```python
from build123d import *

# Parameters (mm, degrees)
SKETCH046_R     = 2.5
PAD023_DEPTH    = 2.5
SKETCH047_R     = 5
PAD024_DEPTH    = 3
FILLET003_R     = 1.5
SKETCH049_R     = 2.5
PAD025_DEPTH    = 4
SKETCH050_R     = 1.5
POCKET026_DEPTH = 4
SKETCH091_W     = 4
SKETCH091_H     = 4
SKETCH091_W_2   = 3
SKETCH091_H_2   = 3
PAD057_DEPTH    = 0.2


with BuildPart() as part:
    # Sketch046 → Pad023 (new body)
    with BuildSketch(Plane(origin=(0, 0, 30), x_dir=(1, 0, 0), z_dir=(0, 0, -1))):
        with Locations((101, 55)):
            Circle(SKETCH046_R)
    extrude(amount=-PAD023_DEPTH)

    # Sketch047 (on Face3 of Pad023) → Pad024 (join)
    with BuildSketch(Plane.XY.offset(32.5)):
        with Locations((101, -55)):
            Circle(SKETCH047_R)
    extrude(amount=PAD024_DEPTH)

    # Fillet003
    fillet003_edges = [part.edges().sort_by_distance(p)[0] for p in [
        (96, -55, 35.5),
    ]]
    fillet(fillet003_edges, radius=FILLET003_R)

    # Sketch049 → Pad025 (join)
    with BuildSketch(Plane(origin=(0, 0, 30), x_dir=(1, 0, 0), z_dir=(0, 0, -1))):
        with Locations((101, 55)):
            Circle(SKETCH049_R)
    extrude(amount=PAD025_DEPTH)

    # Sketch050 (on Face17 of Pad025) → Pocket026 (cut)
    with BuildSketch(Plane(origin=(0, 0, 26), x_dir=(1, 0, 0), z_dir=(0, 0, -1))):
        with Locations((101, 55)):
            Circle(SKETCH050_R)
    extrude(amount=-POCKET026_DEPTH, mode=Mode.SUBTRACT)


with BuildPart() as part_1:
    # Body002 placement: moved
    add(part.part.moved(Location((75, 0, 0))))

    # Sketch091 (on Face4 of Clone005) → Pad057 (new body)
    with BuildSketch(Plane(origin=(75, 0, 35.5), x_dir=(1, 0, 0), z_dir=(0, 0, 1))):
        with Locations((101, -55)):
            Rectangle(SKETCH091_W, SKETCH091_H)
        with Locations((101, -55)):
            Rectangle(SKETCH091_W_2, SKETCH091_H_2, mode=Mode.SUBTRACT)
    extrude(amount=PAD057_DEPTH)


with BuildPart() as part_2:
    # Body014 placement: moved
    add(part_1.part.moved(Location((-64.5, 33.5, 0))))


solid = part_2.part
```
Model file for the job. Use its own axes, mm. A direction names the side the tool comes from. Give positions to 0.01 mm unless a question says otherwise; leave off trailing zeros. Loops run counter-clockwise (first coordinate to the right, second up) from the corner with the lowest first, then second, coordinate; pieces in that order, holes last. Notation, with made-up numbers: (34.25, 41) - (69.25, 41) arc R19 ccw to (69.25, 72) - close; hole circle Ø5 at (77.25, 50). An arc over 180 degrees is marked (long way). One line per item, written item: value. Start each with the question number.
1. Probe L1, parallel to X at y = -21.5, z = 28.2; L2, parallel to Y at x = 111.5, z = 28.2; L3, parallel to Z at x = 110.25, y = -20.75. List the from-to ranges inside material, lowest first. Write a range as from..to.
2. Pin check, flat tips, straight feed: pin 1 (4 mm diameter, centred on y = -25, z = 34, fed in from -X); pin 2 (1.5 mm diameter, centred on y = -18, z = 27, fed in from -X); pin 3 (1 mm diameter, centred on y = -23.5, z = 31.5, fed in from +X); pin 4 (0.9 mm diameter, centred on x = 112, y = -21, fed in from +Z). Stop position of each tip, or through.
3. Slice it at A-A (y = -21.5). List the corners of the cut face in (x, z).
4. Which spindle directions (+Z, -Z, +X, -X, +Y, -Y) get a long thin tool onto all of the face, cutting with end or side? Do faces 1 (the flat face through (113, -20, 26)), 2 (the flat face through (111, -21, 35.5)), 3 (the cylindrical face through (110, -21.57, 27.97)). Say none if no direction does.
5. Slice it at D-D (z = 31.25). List the corners of the cut face in (x, y).
6. Pull direction Y, two halves, no side cores. Call faces 4 (the flat face through (111, -22, 30)), 5 (the flat face through (109.7, -21.5, 35.7)), 6 (the cylindrical face through (116.119, -23.415, 33.24)): pulls with the +Y half, pulls with the -Y half, needs draft (parallel to the pull), parting line crosses it, or undercut.
7. Slice it at C-C (z = 27). List the corners of the cut face in (x, y), plus the area to 3 significant figures.
8. Slice it at B-B (x = 111.5). List the corners of the cut face in (y, z), plus the area to 3 significant figures.
Solution:
1. L1: x = 109..110, 113..114
1. L2: y = -24..-23, -20..-19
1. L3: z = 30..35.5
2. pin 1: stops at x = 106.73
2. pin 2: passes through
2. pin 3: stops at x = 113.5
2. pin 4: stops at z = 35.5
3. outline: (106.5, 32.5) - (109, 32.5) - (109, 26) - (110, 26) - (110, 30) - (113, 30) - (113, 26) - (114, 26) - (114, 32.5) - (116.5, 32.5) - (116.5, 34) arc R1.5 ccw to (115, 35.5) - (113.5, 35.5) - (113.5, 35.7) - (113, 35.7) - (113, 35.5) - (110, 35.5) - (110, 35.7) - (109.5, 35.7) - (109.5, 35.5) - (108, 35.5) arc R1.5 ccw to (106.5, 34) - close
4. face 1: -Z, +X, -X, +Y, -Y
4. face 2: +Z
4. face 3: -Z
5. outline: circle Ø5 at (111.5, -21.5)
6. face 4: undercut
6. face 5: needs draft
6. face 6: parting line crosses it
7. outline: circle Ø5 at (111.5, -21.5); hole circle Ø3 at (111.5, -21.5)
7. area: 12.6 mm^2
8. outline: (-26.5, 32.5) - (-24, 32.5) - (-24, 26) - (-23, 26) - (-23, 30) - (-20, 30) - (-20, 26) - (-19, 26) - (-19, 32.5) - (-16.5, 32.5) - (-16.5, 34) arc R1.5 ccw to (-18, 35.5) - (-19.5, 35.5) - (-19.5, 35.7) - (-20, 35.7) - (-20, 35.5) - (-23, 35.5) - (-23, 35.7) - (-23.5, 35.7) - (-23.5, 35.5) - (-25, 35.5) arc R1.5 ccw to (-26.5, 34) - close
8. area: 49.7 mm^2
